from build123d import *

# Parameters (mm, degrees)
F3_D           = 60.325
F3_CBORE_D     = 60.325
F3_CBORE_DEPTH = 4.826


with BuildPart() as f1:
    # F0 (on Front) → F1 (revolve)
    with BuildSketch(Plane.XZ):
        with BuildLine():
            Line((0, 184.3925616264), (0, 1251.1925616264))
            Line((0, 1251.1925616264), (-254, 1251.1925616264))
            Line((-254, 1251.1925616264), (-254, 1213.0925616264))
            add(Edge.make_bspline(
                [(-254, 1213.0925616264), (-264.7863300499, 1186.664170065), (-288.7208143023, 1128.0205054709), (-299.0989058542, 1043.5793898388), (-304.8, 997.1925616264)],
                knots=[0, 0, 0, 0, 0.4506606424, 1, 1, 1, 1], degree=3))
            Line((-304.8, 997.1925616264), (-304.8, 203.2))
            add(Edge.make_bspline(
                [(-254, 0), (-264.8896198837, 28.1579660638), (-288.0059983927, 87.9314208331), (-298.9902100194, 163.3234862316), (-304.8, 203.2)],
                knots=[0, 0, 0, 0, 0.4710781094, 1, 1, 1, 1], degree=3))
            Line((-254, 0), (0, 0))
            Line((0, 0), (0, 184.3925616264))
        make_face()
    revolve(axis=Axis((0, 0, 717.7925616264), (0, 0, -1)))

    # F3 (through all)
    with Locations(Plane(origin=(0, 0, 0), x_dir=(1, 0, 0), z_dir=(0, 0, -1))):
        with Locations((0, 0)):
            CounterBoreHole(F3_D / 2, F3_CBORE_D / 2, F3_CBORE_DEPTH)


solid = f1.part
Check sheet for the modelled part. Datum: model origin and axes. Units: mm. A direction names the side the tool comes from. Give positions to 0.01 mm unless a question says otherwise; leave off trailing zeros. Write each loop counter-clockwise with the first axis right and the second up, starting at its lowest first coordinate (ties: lowest second). Pieces come first, ordered by that corner, then holes. Notation, with made-up numbers: M 27.5,-1 L 69.5,-1 A9 ccw 69.5,4 Z; hole C 22,51.25 d1. An arc over 180 degrees is marked long. Use one line per item in the form item = value.
(1) Section check A-A on z = 446.5. Record the boundary of the cut face in (x, y) (1 decimal).
Answer block:
outline = C 0,0 d609.6; hole C 0,0 d60.3
(2) Tool access check on faces 1 (the cylindrical face through (55.06, -247.96, 1231.88)), 2 (the flat face through (53, 4, 1251.193)). Record the directions out of +Z, -Z, +X, -X, +Y, -Y that give a thin tool (end or side, any length) a straight path to the whole face; none if there is none.
Answer block:
face_1 = +Z
face_2 = +Z, +X, -X, +Y, -Y
(3) Material ranges on line 1 along Y through (x, z) = (0, 330.5); line 2 along Y through (x, z) = (-20, 992); line 3 along X through (y, z) = (26, 798), recorded low to high.
Answer block:
line_1 = -304.8 to -30.16, 30.16 to 304.8
line_2 = -304.14 to -22.58, 22.58 to 304.14
line_3 = -303.69 to -15.29, 15.29 to 303.69
(4) Depth check by flat-ended pin: P1, Ø5, axis at y = 102, z = 181, coming from the -X side; P2, Ø6, axis at y = 210, z = 650.5, coming from the +X side; P3, Ø8, axis at x = 81.5, z = 286, coming from the +Y side. Enter the tip coordinate at first touch or a pass-through.
Answer block:
P1 = -284.74
P2 = 223.73
P3 = 294.78
